from build123d import *

# Parameters (mm, degrees)
EXTRUDE_1_DEPTH     = 30
CUT_EXTRUDE_1_DEPTH = 98
SKETCH_3_W          = 46
SKETCH_3_H          = 11.7
CUT_EXTRUDE_2_DEPTH = 25
SKETCH_4_W          = 33.079477917
SKETCH_4_H          = 22.974752345
CUT_EXTRUDE_3_DEPTH = 46


with BuildPart() as part:
    # Эскиз1 → Бобышка-Вытянуть1 (new body)
    with BuildSketch(Plane(origin=(0, 0, 0), x_dir=(1, 0, 0), z_dir=(0, 1, 0))):
        Polygon((-49, 100), (49, 100), (49, 32), (23, 32), (23, 2), (-23, 2), (-23, 32), (-49, 32), align=None)
    extrude(amount=EXTRUDE_1_DEPTH)

    # Эскиз2 → Вырез-Вытянуть1 (cut)
    with BuildSketch(Plane.ZY.offset(49)):
        Polygon((-99, 0), (-54, 30), (-54, 44.902794758), (-113.255457038, 44.902794758), (-113.255457038, 0), align=None)
    extrude(amount=-CUT_EXTRUDE_1_DEPTH, mode=Mode.SUBTRACT)

    # Эскиз3 → Вырез-Вытянуть2 (cut)
    with BuildSketch(Plane(origin=(0, 30, 0), x_dir=(1, 0, 0), z_dir=(0, 1, 0))):
        with Locations((0, 16)):
            Rectangle(SKETCH_3_W, SKETCH_3_H)
    extrude(amount=-CUT_EXTRUDE_2_DEPTH, mode=Mode.SUBTRACT)

    # Эскиз4 → Вырез-Вытянуть3 (cut)
    with BuildSketch(Plane.ZY.offset(23)):
        with Locations((-15.460261042, 20.487376172)):
            Rectangle(SKETCH_4_W, SKETCH_4_H)
    extrude(amount=-CUT_EXTRUDE_3_DEPTH, mode=Mode.SUBTRACT)


solid = part.part
Build history of the part. All positions in model axes, mm. A direction names the side the tool comes from. Round coordinates to 2 decimals unless told otherwise and drop trailing zeros. Write each loop counter-clockwise with the first axis right and the second up, starting at its lowest first coordinate (ties: lowest second). Pieces come first, ordered by that corner, then holes. Notation, with made-up numbers: (-1.5, 46) -> (53.5, 46) arc R20 ccw to (53.5, 66) -> close; hole circle Ø1 at (72.5, 69). An arc over 180 degrees is marked (long way). Use one line per item in the form item = value.
Q1. Drop flat-ended pins along their axis: P1, Ø3, axis at x = -29, z = -31.5, coming from the -Y side; P2, Ø2, axis at x = 10, y = 8, coming from the -Z side; P3, Ø7, axis at y = 4, z = -23, coming from the +X side; P4, Ø9.5, axis at x = 9.5, z = -18, coming from the +Y side. Give the stop position or say it passes through.
Conclusion:
P1 = 0
P2 = -88.5
P3 = 23
P4 = 9
Q2. Band-saw the part on B-B, the plane x = 5.5. Write the cut outline in (y, z), then the cut area to 3 significant figures.
Conclusion:
outline = (0, -99) -> (30, -54) -> (30, -32) -> (9, -32) -> (9, -21.85) -> (5, -21.85) -> (5, -10.15) -> (9, -10.15) -> (9, -2) -> (0, -2) -> close
area = 1,560 mm²
Q3. Two-plate mould, pull along Z, no slides. Class faces 1 (the flat face through (-0.7, 14.8, -76.8)), 2 (the flat face through (0, 9, -27)), 3 (the flat face through (0, 5, -16)): released by +Z, released by -Z, zero draft, split by the parting line, or undercut.
Conclusion:
face_1 = released by -Z
face_2 = zero draft
face_3 = undercut
Q4. Tool access for faces 4 (the flat face through (-23, 4, -17)), 5 (the flat face through (1, 0, -62)), 6 (the flat face through (0, 9, -6)), 7 (the flat face through (23, 3, -17)), 8 (the flat face through (0, 7, -21.85)): list every direction of +Z, -Z, +X, -X, +Y, -Y with a clear straight run to the whole face (end or side of a thin tool).
Conclusion:
face_4 = +Z, -X, +Y, -Y
face_5 = +Z, -Z, +X, -X, -Y
face_6 = +Z, +X, -X, +Y
face_7 = +Z, +X, +Y, -Y
face_8 = +X, -X, +Y
Q5. Band-saw the part on A-A, the plane y = 2. Write the cut outline in (x, z), then the cut area to 3 significant figures.
Conclusion:
outline = (-49, -96) -> (49, -96) -> (49, -32) -> (23, -32) -> (23, -2) -> (-23, -2) -> (-23, -32) -> (-49, -32) -> close
area = 7,650 mm²
Q6. Drill centre lines: L1, parallel to Y at x = -25.5, z = -71.5; L2, parallel to Y at x = 31.5, z = -60; L3, parallel to Z at x = 7.5, y = 8.25 (3 decimals). Where is each one in solid material? Low to high.
Conclusion:
L1 = 0 to 18.33
L2 = 0 to 26
L3 = -86.625 to -21.85, -10.15 to -2
Q7. Band-saw the part on C-C, the plane z = -9. Write the cut outline in (x, y).
Conclusion:
outline = (-23, 0) -> (23, 0) -> (23, 9) -> (-23, 9) -> close
Q8. Band-saw the part on D-D, the plane y = 20.5. Write the cut outline in (x, z).
Conclusion:
outline = (-49, -68.25) -> (49, -68.25) -> (49, -32) -> (-49, -32) -> close
